```python
from build123d import *

# Parameters (mm, degrees)
SKETCH1_R               = 35.56
BOSS_EXTRUDE1_DEPTH     = 3.25
SKETCH2_R               = 9.5
CUT_EXTRUDE1_DEPTH      = 51.707762719
CIRPATTERN1_COUNT       = 6
SKETCH3_R               = 2.25
CUT_EXTRUDE2_DEPTH      = 3
CIRPATTERN2_COUNT       = 3
CUT_EXTRUDE3_DEPTH      = 51.261210864
CUT_EXTRUDE3_DEPTH_BACK = 51.261210864
SKETCH4_R               = 2.25
SKETCH5_R               = 2
BOSS_EXTRUDE2_DEPTH     = 2.5
CIRPATTERN3_COUNT       = 3
CUT_EXTRUDE4_DEPTH      = 51.261210864


with BuildPart() as part:
    # Sketch1 → Boss-Extrude1 (new, symmetric)
    with BuildSketch(Plane(origin=(0, 0, 0), x_dir=(1, 0, 0), z_dir=(0, 1, 0))):
        with Locations(Location((0, 0, 0), (0, 0, 90))):
            Circle(SKETCH1_R)
    extrude(amount=BOSS_EXTRUDE1_DEPTH, both=True)

    # Sketch2 → Cut-Extrude1 (cut, through all)
    with BuildSketch(Plane(origin=(0, 3.25, 0), x_dir=(1, 0, 0), z_dir=(0, 1, 0))):
        with Locations((0, 28.2)):
            Circle(SKETCH2_R)
    cut_extrude1 = extrude(amount=-CUT_EXTRUDE1_DEPTH, mode=Mode.SUBTRACT)

    # CirPattern1: Cut-Extrude1 ×6 about axis
    cirpattern1_axis = Axis((0, 0, 0), (0, 1, 0))
    for i in range(1, CIRPATTERN1_COUNT):
        add(cut_extrude1.rotate(cirpattern1_axis, i * 360 / CIRPATTERN1_COUNT), mode=Mode.SUBTRACT)

    # Sketch3 → Cut-Extrude2 (cut)
    with BuildSketch(Plane(origin=(0, 3.25, 0), x_dir=(1, 0, 0), z_dir=(0, 1, 0))):
        with Locations(Location((0, 10, 0), (0, 0, 270))):
            Circle(SKETCH3_R)
    cut_extrude2 = extrude(amount=-CUT_EXTRUDE2_DEPTH, mode=Mode.SUBTRACT)

    # CirPattern2: Cut-Extrude2 ×3 about axis
    cirpattern2_axis = Axis((0, 0, 0), (0, 1, 0))
    for i in range(1, CIRPATTERN2_COUNT):
        add(cut_extrude2.rotate(cirpattern2_axis, i * 360 / CIRPATTERN2_COUNT), mode=Mode.SUBTRACT)

    # Sketch4 → Cut-Extrude3 (cut, two sides: drawn at the far end of the back side and taken through both)
    with BuildSketch(Plane(origin=(0, 3.25, 0), x_dir=(1, 0, 0), z_dir=(0, 1, 0)).offset(-CUT_EXTRUDE3_DEPTH_BACK)):
        with Locations(Location((0, 0, 0), (0, 0, 270))):
            Circle(SKETCH4_R)
    extrude(amount=CUT_EXTRUDE3_DEPTH + CUT_EXTRUDE3_DEPTH_BACK, mode=Mode.SUBTRACT)

    # Sketch5 → Boss-Extrude2 (add)
    with BuildSketch(Plane(origin=(0, -3.25, 0), x_dir=(-1, 0, 0), z_dir=(0, -1, 0))):
        with Locations(Location((0, 10, 0), (0, 0, 270))):
            Circle(SKETCH5_R)
    boss_extrude2 = extrude(amount=BOSS_EXTRUDE2_DEPTH)

    # CirPattern3: Boss-Extrude2 ×3 about axis
    cirpattern3_axis = Axis((0, 0, 0), (0, 1, 0))
    for i in range(1, CIRPATTERN3_COUNT):
        add(boss_extrude2.rotate(cirpattern3_axis, i * 360 / CIRPATTERN3_COUNT))

    # Sketch6 → Cut-Extrude4 (cut, through all)
    with BuildSketch(Plane.XZ.offset(3.25)):
        Polygon((-12.047949192, 24.867660128), (-15.512050808, 22.867660128), (-19.512050808, 29.795863359), (-16.047949192, 31.795863359), align=None)
    extrude(amount=-CUT_EXTRUDE4_DEPTH, mode=Mode.SUBTRACT)


solid = part.part
```
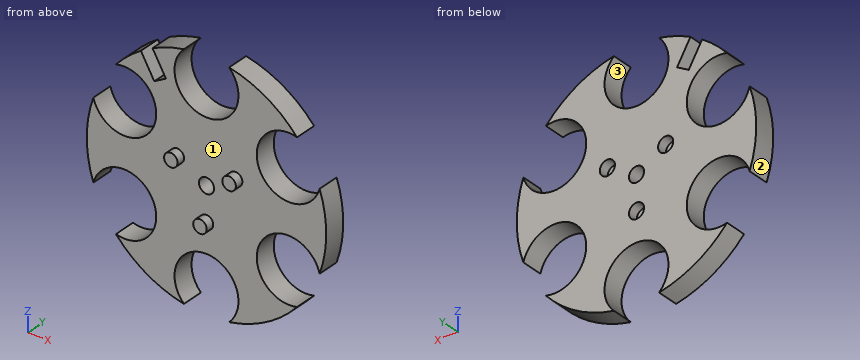
Part model, mm, in its own coordinate system. Face numbers are marked on the shaded views. Round coordinates to 2 decimals unless told otherwise and drop trailing zeros. Order: outer loops, then holes, each group sorted by start corner. A loop starts at its lowest first (then second) coordinate and runs counter-clockwise, first axis right, second up. Notation, with made-up numbers: M 80,83.25 L 112,83.25 A18 ccw 112,94.25 Z; hole C 46,-18 d2. An arc over 180 degrees is marked long. Answer in a Markdown table with one row per item. Add a question column.
Q1. Wall check: L1, parallel to X at y = 1, z = 28.2; L2, parallel to Z at x = -20.5, y = 1.75; L3, parallel to X at y = 0, z = 6.5. Give the ranges that are in metal, low to high. Write a range as from..to.
Q2. Cut at C-C on z = 0. Give the cut face in (x, y).
Q3. Cut at B-B on y = -0.75. Give the cut face in (x, z) (3 decimals), and give its area (3 significant figures).
Q4. Mould opens along Z. For the marked faces 1, 2 and 3 say: +Z half, -Z half, draft (parallel to the pull), parting line (faces both ways), or undercut.
Q5. Pin check, flat tips, straight feed: pin 1 (4 mm diameter, centred on x = -12, z = -27.5, fed in from -Y); pin 2 (3.5 mm diameter, centred on x = 9.5, z = 4, fed in from +Y); pin 3 (4 mm diameter, centred on y = -1, z = -3.5, fed in from -X); pin 4 (1.5 mm diameter, centred on y = 1, z = 14.5, fed in from -X). Stop position of each tip, or through.
Q6. Cut at D-D on z = 28.2. Give the cut face in (x, y).
Q7. Cut at A-A on x = 0. Give the cut face in (y, z), and give its area (3 significant figures).
Established:
| question | item | result |
|---|---|---|
| 1 | L1 | x = -21.66..-18.59, -13.97..-9.5, 9.5..21.66 |
| 1 | L2 | z = -29.06..-22.75, -5.45..5.45, 22.75..29.06 |
| 1 | L3 | x = -34.96..-30.12, -18.72..18.72, 30.12..34.96 |
| 2 | outline | M -35.56,-3.25 L -2.25,-3.25 L -2.25,3.25 L -35.56,3.25 Z; M 2.25,-3.25 L 35.56,-3.25 L 35.56,3.25 L 2.25,3.25 Z |
| 3 | outline | M -33.599,-11.645 A9.5 cw long -26.884,-23.275 A35.56 ccw -6.715,-34.92 A9.5 cw long 6.715,-34.92 A35.56 ccw 26.884,-23.275 A9.5 cw long 33.599,-11.645 A35.56 ccw 33.599,11.645 A9.5 cw long 26.884,23.275 A35.56 ccw 6.715,34.92 A9.5 cw long -6.715,34.92 A35.56 ccw -16.02,31.747 L -12.048,24.868 L -15.512,22.868 L -19.484,29.747 A35.56 ccw -26.884,23.275 A9.5 cw long -33.599,11.645 A35.56 ccw Z; hole C 0,0 d4.5 |
| 3 | area | 2,340 mm2 |
| 4 | face 1 | draft |
| 4 | face 2 | parting line |
| 4 | face 3 | undercut |
| 5 | pin 1 | stops at y = -3.25 |
| 5 | pin 2 | stops at y = 3.25 |
| 5 | pin 3 | stops at x = -35.53 |
| 5 | pin 4 | stops at x = -14.99 |
| 6 | outline | M -21.66,-3.25 L -18.59,-3.25 L -18.59,3.25 L -21.66,3.25 Z; M -13.97,-3.25 L -9.5,-3.25 L -9.5,3.25 L -13.97,3.25 Z; M 9.5,-3.25 L 21.66,-3.25 L 21.66,3.25 L 9.5,3.25 Z |
| 7 | outline | M -5.75,-12 L -3.25,-12 L -3.25,-18.7 L 3.25,-18.7 L 3.25,-12.25 L 0.25,-12.25 L 0.25,-7.75 L 3.25,-7.75 L 3.25,-2.25 L -3.25,-2.25 L -3.25,-8 L -5.75,-8 Z; M -3.25,2.25 L 3.25,2.25 L 3.25,18.7 L -3.25,18.7 Z |
| 7 | area | 210 mm2 |
